Model file for the job. Use its own axes, mm. Round coordinates to 2 decimals unless told otherwise and drop trailing zeros. Order: outer loops, then holes, each group sorted by start corner. A loop starts at its lowest first (then second) coordinate and runs counter-clockwise, first axis right, second up. Notation, with made-up numbers: (18, 50.5) -> (53, 50.5) arc R23 ccw to (53, 82.5) -> close; hole circle Ø11 at (84.5, -38.75). An arc over 180 degrees is marked (long way). Answer as CSV lines item,"result".
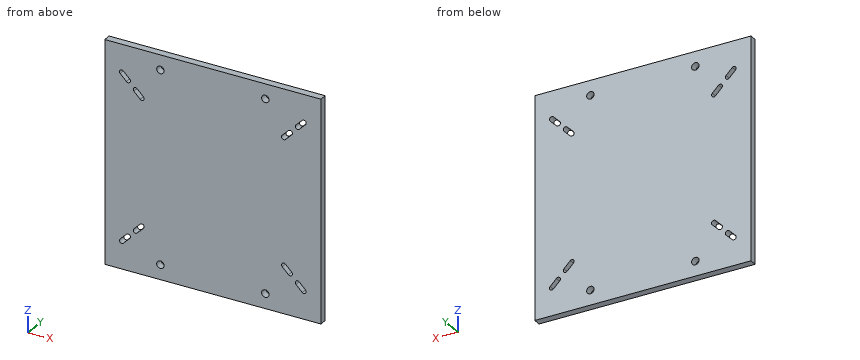
```python
from build123d import *

# Parameters (mm, degrees)
SKETCH1_W              = 185.4
SKETCH1_H              = 190
BASE_PLATE_DEPTH       = 6.35
SLOTS_DEPTH            = 7.35
FEET_CONNECTION_HOLE_D = 6.35


with BuildPart() as part:
    # Sketch1 → base plate (new body)
    with BuildSketch(Plane(origin=(0, 0, 0), x_dir=(1, 0, 0), z_dir=(0, 1, 0))):
        with Locations((92.7, -95)):
            Rectangle(SKETCH1_W, SKETCH1_H)
    extrude(amount=-BASE_PLATE_DEPTH)

    # Sketch3 → slots (cut, through all)
    with BuildSketch(Plane(origin=(0, 0, 0), x_dir=(1, 0, 0), z_dir=(0, 1, 0))):
        with BuildLine():
            ThreePointArc((21.424612456, -27.64618524), (21.424612456, -30.474612456), (18.59618524, -30.474612456))
            Line((18.59618524, -30.474612456), (13.208031568, -25.086458783))
            ThreePointArc((13.208031568, -25.086458783), (13.208031568, -22.258031568), (16.036458783, -22.258031568))
            Line((16.036458783, -22.258031568), (21.424612456, -27.64618524))
        make_face()
        with BuildLine():
            Line((169.363541217, -22.258031568), (163.975387544, -27.64618524))
            ThreePointArc((163.975387544, -27.64618524), (163.975387544, -30.474612456), (166.80381476, -30.474612456))
            Line((166.80381476, -30.474612456), (172.191968432, -25.086458783))
            ThreePointArc((172.191968432, -25.086458783), (172.191968432, -22.258031568), (169.363541217, -22.258031568))
        make_face()
        with BuildLine():
            Line((154.995131423, -42.283295792), (160.383285096, -36.895142119))
            ThreePointArc((160.383285096, -36.895142119), (160.383285096, -34.066714904), (157.554857881, -34.066714904))
            Line((157.554857881, -34.066714904), (152.166704208, -39.454868577))
            ThreePointArc((152.166704208, -39.454868577), (152.166704208, -42.283295792), (154.995131423, -42.283295792))
        make_face()
        with BuildLine():
            ThreePointArc((160.383285096, -153.104857881), (160.383285096, -155.933285096), (157.554857881, -155.933285096))
            Line((157.554857881, -155.933285096), (152.166704208, -150.545131423))
            ThreePointArc((152.166704208, -150.545131423), (152.166704208, -147.716704208), (154.995131423, -147.716704208))
            Line((154.995131423, -147.716704208), (160.383285096, -153.104857881))
        make_face()
        with BuildLine():
            ThreePointArc((163.975387544, -162.35381476), (163.975387544, -159.525387544), (166.80381476, -159.525387544))
            Line((166.80381476, -159.525387544), (172.191968432, -164.913541217))
            ThreePointArc((172.191968432, -164.913541217), (172.191968432, -167.741968432), (169.363541217, -167.741968432))
            Line((169.363541217, -167.741968432), (163.975387544, -162.35381476))
        make_face()
        with BuildLine():
            Line((16.036458783, -167.741968432), (21.424612456, -162.35381476))
            ThreePointArc((21.424612456, -162.35381476), (21.424612456, -159.525387544), (18.59618524, -159.525387544))
            Line((18.59618524, -159.525387544), (13.208031568, -164.913541217))
            ThreePointArc((13.208031568, -164.913541217), (13.208031568, -167.741968432), (16.036458783, -167.741968432))
        make_face()
        with BuildLine():
            Line((30.404868577, -147.716704208), (25.016714904, -153.104857881))
            ThreePointArc((25.016714904, -153.104857881), (25.016714904, -155.933285096), (27.845142119, -155.933285096))
            Line((27.845142119, -155.933285096), (33.233295792, -150.545131423))
            ThreePointArc((33.233295792, -150.545131423), (33.233295792, -147.716704208), (30.404868577, -147.716704208))
        make_face()
        with BuildLine():
            Line((30.404868577, -42.283295792), (25.016714904, -36.895142119))
            ThreePointArc((25.016714904, -36.895142119), (25.016714904, -34.066714904), (27.845142119, -34.066714904))
            Line((27.845142119, -34.066714904), (33.233295792, -39.454868577))
            ThreePointArc((33.233295792, -39.454868577), (33.233295792, -42.283295792), (30.404868577, -42.283295792))
        make_face()
    extrude(amount=-SLOTS_DEPTH, mode=Mode.SUBTRACT)

    # Feet connection hole (through all)
    with Locations(Plane(origin=(0, 0, 0), x_dir=(1, 0, 0), z_dir=(0, 1, 0))):
        with Locations((47.7, -177.3), (137.7, -12.7), (47.7, -12.7), (137.7, -177.3)):
            Hole(FEET_CONNECTION_HOLE_D / 2)


solid = part.part
```
Q1. Saw through at B-B (z = 12.7). Write the cut outline in (x, y) (3 decimals), plus the area to 3 significant figures.
Checks:
outline,"(0, -6.35) -> (44.525, -6.35) -> (44.525, 0) -> (0, 0) -> close; (50.875, -6.35) -> (134.525, -6.35) -> (134.525, 0) -> (50.875, 0) -> close; (140.875, -6.35) -> (185.4, -6.35) -> (185.4, 0) -> (140.875, 0) -> close"
area,"1,100 mm²"
Q2. Saw through at A-A (x = 137.7). Write the cut outline in (y, z) (3 decimals).
Checks:
outline,"(-6.35, 0) -> (0, 0) -> (0, 9.525) -> (-6.35, 9.525) -> close; (-6.35, 15.875) -> (0, 15.875) -> (0, 174.125) -> (-6.35, 174.125) -> close; (-6.35, 180.475) -> (0, 180.475) -> (0, 190) -> (-6.35, 190) -> close"
Q3. Flat gauge pin, fed straight in: pin 1 (4 mm diameter, centred on x = 137.7, z = 177.3, fed in from +Y). Where does the tip first touch, or does it go through?
Checks:
pin 1,"through"
Q4. Wall check: L1, parallel to X at y = -4.25, z = 12.7 (3 decimals); L2, parallel to Z at x = 47.7, y = -3.25 (3 decimals); L3, parallel to Z at x = 139.5, y = -4. Give the ranges that are in metal, low to high. Write a range as [from, to].
Checks:
L1,"[0, 44.525], [50.875, 134.525], [140.875, 185.4]"
L2,"[0, 9.525], [15.875, 174.125], [180.475, 190]"
L3,"[0, 10.08], [15.32, 174.68], [179.92, 190]"
